The figure shows three views and two pictorial views of one solid part (mm, origin at its lowest corner). Answer the questions. Coordinates: 2 decimals unless noted, no trailing zeros. Order: outer loops, then holes, each group sorted by start corner. A loop starts at its lowest first (then second) coordinate and runs counter-clockwise, first axis right, second up. Notation, with made-up numbers: (56, 38) -> (80, 38) arc R17 cw to (80, 45) -> close; hole circle Ø7 at (50, 89.25). An arc over 180 degrees is marked (long way). Return JSON: item names as keys, results as strings.
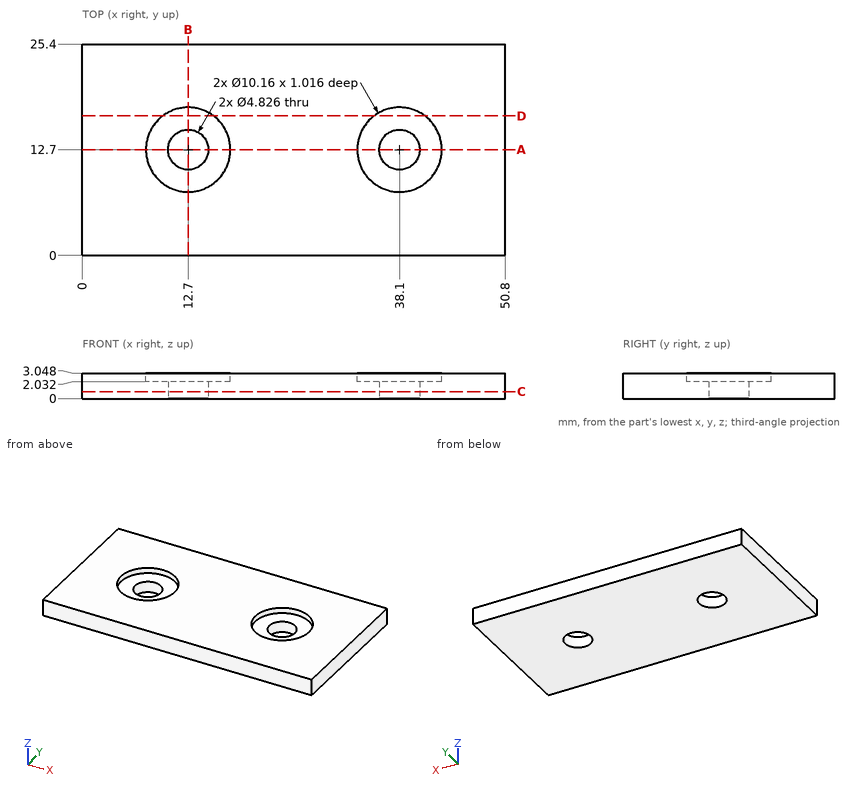
Item 1: A flat-ended cylindrical pin translates along its axis: pin 1 (7.5 mm diameter, centred on x = 38.1, y = 12.7, fed in from +Z). Find the tip coordinate at first contact, or state that the pin passes through.
Answer list:
{"pin 1": "z = 2.03"}
Item 2: The part is cut by section A-A on y = 12.7. Determine the outline of the cut face in (x, z), plus the area to 3 significant figures.
Answer list:
{"outline": "(0, 0) -> (10.29, 0) -> (10.29, 2.03) -> (7.62, 2.03) -> (7.62, 3.05) -> (0, 3.05) -> close; (15.11, 0) -> (35.69, 0) -> (35.69, 2.03) -> (33.02, 2.03) -> (33.02, 3.05) -> (17.78, 3.05) -> (17.78, 2.03) -> (15.11, 2.03) -> close; (40.51, 0) -> (50.8, 0) -> (50.8, 3.05) -> (43.18, 3.05) -> (43.18, 2.03) -> (40.51, 2.03) -> close", "area": "115 mm2"}
Item 3: The part is cut by section D-D on y = 16.75. Determine the outline of the cut face in (x, z).
Answer list:
{"outline": "(0, 0) -> (50.8, 0) -> (50.8, 3.05) -> (41.17, 3.05) -> (41.17, 2.03) -> (35.03, 2.03) -> (35.03, 3.05) -> (15.77, 3.05) -> (15.77, 2.03) -> (9.63, 2.03) -> (9.63, 3.05) -> (0, 3.05) -> close"}
Item 4: The part is cut by section B-B on x = 12.7. Determine the outline of the cut face in (y, z), plus the area to 3 significant figures.
Answer list:
{"outline": "(0, 0) -> (10.29, 0) -> (10.29, 2.03) -> (7.62, 2.03) -> (7.62, 3.05) -> (0, 3.05) -> close; (15.11, 0) -> (25.4, 0) -> (25.4, 3.05) -> (17.78, 3.05) -> (17.78, 2.03) -> (15.11, 2.03) -> close", "area": "57.3 mm2"}
Item 5: The part is cut by section C-C on z = 0.85. Determine the outline of the cut face in (x, y), plus the area to 3 significant figures.
Answer list:
{"outline": "(0, 0) -> (50.8, 0) -> (50.8, 25.4) -> (0, 25.4) -> close; hole circle Ø4.83 at (12.7, 12.7); hole circle Ø4.83 at (38.1, 12.7)", "area": "1,250 mm2"}
Item 6: Find the intervals of material crossed by probe 1 along X at (y, z) = (12.5, 1.2); probe 2 along Y at (x, z) = (12.7, 1.5); probe 3 along X at (y, z) = (10.5, 0.7), in increasing order.
Answer list:
{"probe 1": "0 to 10.3, 15.1 to 35.7, 40.5 to 50.8", "probe 2": "0 to 10.29, 15.11 to 25.4", "probe 3": "0 to 11.71, 13.69 to 37.11, 39.09 to 50.8"}
